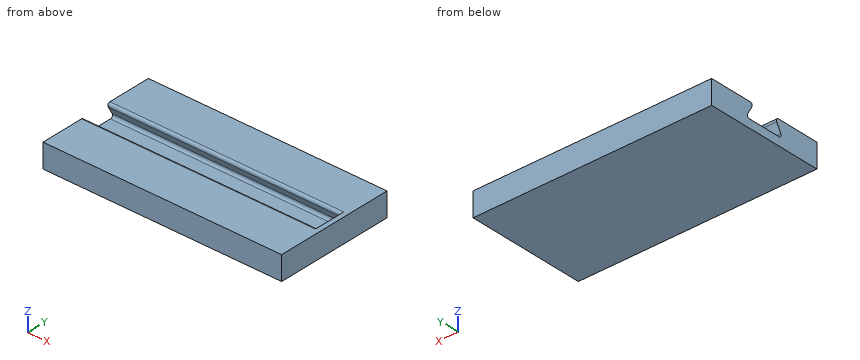
from build123d import *

# Parameters (mm, degrees)
IZIM1_W                     = 100
IZIM1_H                     = 50
Y_KSEKLIK_EKSTR_ZYON1_DEPTH = 10
KES_EKSTR_ZYON1_DEPTH       = 98
RADYUS1_R                   = 1


with BuildPart() as part:
    # Çizim1 → Yükseklik-Ekstrüzyon1 (new body)
    with BuildSketch(Plane.XY):
        Rectangle(IZIM1_W, IZIM1_H)
    extrude(amount=Y_KSEKLIK_EKSTR_ZYON1_DEPTH)

    # Çizim2 → Kes-Ekstrüzyon1 (cut)
    with BuildSketch(Plane.ZY.offset(50)):
        Polygon((10, 5), (3.504809472, 8.75), (3.504809472, -8.75), (10, -5), align=None)
    extrude(amount=-KES_EKSTR_ZYON1_DEPTH, mode=Mode.SUBTRACT)

    # Radyus1
    radyus1_edges = [part.edges().sort_by_distance(p)[0] for p in [
        (-1, 5, 10),
        (-1, -5, 10),
        (-1, -8.75, 3.504809472),
        (-1, 8.75, 3.504809472),
    ]]
    fillet(radyus1_edges, radius=RADYUS1_R)


solid = part.part
Design review of the part built by this model. Coordinates are the model's own, in mm. Give positions to 0.01 mm unless a question says otherwise; leave off trailing zeros. Loops run counter-clockwise (first coordinate to the right, second up) from the corner with the lowest first, then second, coordinate; pieces in that order, holes last. Notation, with made-up numbers: (30, 62) - (39, 62) arc R22 cw to (39, 100) - close; hole circle Ø4 at (24, 23). An arc over 180 degrees is marked (long way). Write item = value, one per line.
1) Take a section at B-B on z = 6. State the section outline as (x, y) points.
Result sheet:
outline = (-50, -25) - (50, -25) - (50, 25) - (-50, 25) - (-50, 7.31) - (48, 7.31) - (48, -7.31) - (-50, -7.31) - close
2) Take a section at C-C on y = -4. State the section outline as (x, z) points, and give its area (3 significant figures).
Result sheet:
outline = (-50, 0) - (50, 0) - (50, 10) - (48, 10) - (48, 3.5) - (-50, 3.5) - close
area = 363 mm2
3) Take a section at A-A on x = 21.5. State the section outline as (y, z) points.
Result sheet:
outline = (-25, 0) - (25, 0) - (25, 10) - (6.73, 10) arc R1 ccw to (5.87, 8.5) - (7.88, 5) arc R1 cw to (7.02, 3.5) - (-7.02, 3.5) arc R1 cw to (-7.88, 5) - (-5.87, 8.5) arc R1 ccw to (-6.73, 10) - (-25, 10) - close
4) Clearance check with flat-ended pins moving along their axes: pin 1 Ø1.5 at (x, y) = (10.5, 1.5) entering from +Z; pin 2 Ø1.9 at (y, z) = (3.5, 7.5) entering from -X. State where each tip first meets the part, or that it passes through.
Result sheet:
pin_1 = 3.5
pin_2 = 48
5) To check wall thickness, follow line 1 (Y direction, x = 31, z = 8.5); line 2 (Y direction, x = -7, z = 4.5); line 3 (Z direction, x = 24, y = 1.5). State the ranges of each line that lie inside material, in increasing order.
Result sheet:
line_1 = -25 to -5.87, 5.87 to 25
line_2 = -25 to -8.02, 8.02 to 25
line_3 = 0 to 3.5
